Check sheet for the modelled part. Datum: model origin and axes. Units: mm. Give positions to 0.01 mm unless a question says otherwise; leave off trailing zeros. Loops run counter-clockwise (first coordinate to the right, second up) from the corner with the lowest first, then second, coordinate; pieces in that order, holes last. Notation, with made-up numbers: (69, 69) - (79, 69) arc R28 cw to (79, 94) - close; hole circle Ø4 at (35, 77). An arc over 180 degrees is marked (long way). Use CSV: the item, a comma, the result in double quotes.
from build123d import *

# Parameters (mm, degrees)
F1_ANGLE = 180
F2_DEPTH = 2.54
F3_DEPTH = 5.08


with BuildPart() as f1:
    # F0 (on Top) → F1 (revolve)
    with BuildSketch(Plane.XY):
        with BuildLine():
            ThreePointArc((0, -39.37), (-39.37, 0), (0, 39.37))
            Line((0, 39.37), (0, 40.64))
            ThreePointArc((0, 40.64), (-40.64, 0), (0, -40.64))
            Line((0, -40.64), (0, -39.37))
        make_face()
    revolve(axis=Axis((0, 7.1776621044, 0), (0, -1, 0)), revolution_arc=F1_ANGLE)

    # F0 (on Top) → F2 (join)
    with BuildSketch(Plane.XY):
        with BuildLine():
            Line((0, 40.64), (0, 39.37))
            ThreePointArc((0, 39.37), (27.8387939753, 27.8387939753), (39.37, 0))
            ThreePointArc((39.37, 0), (27.8387939753, -27.8387939753), (0, -39.37))
            Line((0, -39.37), (0, -40.64))
            ThreePointArc((0, -40.64), (28.7368195874, -28.7368195874), (40.64, 0))
            ThreePointArc((40.64, 0), (28.7368195874, 28.7368195874), (0, 40.64))
        make_face()
        with BuildLine():
            ThreePointArc((0, 35.2425), (24.920210736, 24.920210736), (35.2425, 0))
            ThreePointArc((35.2425, 0), (24.920210736, -24.920210736), (0, -35.2425))
            Line((0, -35.2425), (0, -37.7825))
            ThreePointArc((0, -37.7825), (26.7162619602, -26.7162619602), (37.7825, 0))
            ThreePointArc((37.7825, 0), (26.7162619602, 26.7162619602), (0, 37.7825))
            Line((0, 37.7825), (0, 35.2425))
        make_face()
        with BuildLine():
            ThreePointArc((0, -39.37), (-39.37, 0), (0, 39.37))
            Line((0, 39.37), (0, 40.64))
            ThreePointArc((0, 40.64), (-40.64, 0), (0, -40.64))
            Line((0, -40.64), (0, -39.37))
        make_face()
        with BuildLine():
            ThreePointArc((0, -35.2425), (-35.2425, 0), (0, 35.2425))
            Line((0, 35.2425), (0, 37.7825))
            ThreePointArc((0, 37.7825), (-37.7825, 0), (0, -37.7825))
            Line((0, -37.7825), (0, -35.2425))
        make_face()
        with BuildLine():
            ThreePointArc((0, -37.7825), (-37.7825, 0), (0, 37.7825))
            Line((0, 37.7825), (0, 39.37))
            ThreePointArc((0, 39.37), (-39.37, 0), (0, -39.37))
            Line((0, -39.37), (0, -37.7825))
        make_face()
        with BuildLine():
            Line((0, 39.37), (0, 37.7825))
            ThreePointArc((0, 37.7825), (26.7162619602, 26.7162619602), (37.7825, 0))
            ThreePointArc((37.7825, 0), (26.7162619602, -26.7162619602), (0, -37.7825))
            Line((0, -37.7825), (0, -39.37))
            ThreePointArc((0, -39.37), (27.8387939753, -27.8387939753), (39.37, 0))
            ThreePointArc((39.37, 0), (27.8387939753, 27.8387939753), (0, 39.37))
        make_face()
    extrude(amount=F2_DEPTH)

    # F0 (on Top) → F3 (join)
    with BuildSketch(Plane.XY):
        with BuildLine():
            ThreePointArc((0, 35.2425), (24.920210736, 24.920210736), (35.2425, 0))
            ThreePointArc((35.2425, 0), (24.920210736, -24.920210736), (0, -35.2425))
            Line((0, -35.2425), (0, -37.7825))
            ThreePointArc((0, -37.7825), (26.7162619602, -26.7162619602), (37.7825, 0))
            ThreePointArc((37.7825, 0), (26.7162619602, 26.7162619602), (0, 37.7825))
            Line((0, 37.7825), (0, 35.2425))
        make_face()
        with BuildLine():
            ThreePointArc((0, -35.2425), (-35.2425, 0), (0, 35.2425))
            Line((0, 35.2425), (0, 37.7825))
            ThreePointArc((0, 37.7825), (-37.7825, 0), (0, -37.7825))
            Line((0, -37.7825), (0, -35.2425))
        make_face()
    extrude(amount=F3_DEPTH)


solid = f1.part
1. Go/stop test with flat-tipped pins: pin 1 Ø10 at (x, y) = (22, 10.5) entering from -Z; pin 2 Ø5 at (y, z) = (-9, -3.5) entering from -X; pin 3 Ø6 at (x, z) = (3.5, -10.5) entering from -Y. Record where each tip stops, or that it passes through.
Completed:
pin 1,"stops at z = -35.72"
pin 2,"stops at x = -40"
pin 3,"stops at y = -39.83"
2. Sectioned sample at C-C, the plane z = -31.5. Record the boundary of the cut face in (x, y), and give its area (3 significant figures).
Completed:
outline,"circle Ø51.36 at (0, 0); hole circle Ø47.23 at (0, 0)"
area,"319 mm²"
3. Sectioned sample at A-A, the plane x = -4. Record the boundary of the cut face in (y, z).
Completed:
outline,"(-40.44, 0) arc R40.44 ccw to (40.44, 0) - (40.44, 2.54) - (37.57, 2.54) - (37.57, 5.08) - (35.01, 5.08) - (35.01, 0) - (39.17, 0) arc R39.17 cw to (-39.17, 0) - (-35.01, 0) - (-35.01, 5.08) - (-37.57, 5.08) - (-37.57, 2.54) - (-40.44, 2.54) - close"
4. Sectioned sample at B-B, the plane y = 16.5. Record the boundary of the cut face in (x, z).
Completed:
outline,"(-37.14, 0) arc R37.14 ccw to (37.14, 0) - (37.14, 2.54) - (33.99, 2.54) - (33.99, 5.08) - (31.14, 5.08) - (31.14, 0) - (35.75, 0) arc R35.75 cw to (-35.75, 0) - (-31.14, 0) - (-31.14, 5.08) - (-33.99, 5.08) - (-33.99, 2.54) - (-37.14, 2.54) - close"
5. Release check for a two-part mould opening along Y. For faces 1 (the face through (-10.586, -33.615, 2.504)), 2 (the face through (-29.3, -20.2, 0)), 3 (the face through (11, 34, 5.08)) record: released by +Y, released by -Y, zero draft, split by the parting line, or undercut.
Completed:
face 1,"undercut"
face 2,"undercut"
face 3,"zero draft"
6. Scan lines: line 1 along Y through (x, z) = (3.5, -31); line 2 along Z through (x, y) = (-25.5, 25); line 3 along Y through (x, z) = (-15.5, -23). Record each from-to range of solid material in increasing order.
Completed:
line 1,"y = -26.05 to -24.02, 24.02 to 26.05"
line 2,"z = -19.4 to -16.58, 0 to 5.08"
line 3,"y = -29.7 to -27.94, 27.94 to 29.7"
